The model under review builds one solid part; all positions refer to its coordinate system, in mm. A direction names the side the tool comes from. Round coordinates to 2 decimals unless told otherwise and drop trailing zeros. Order: outer loops, then holes, each group sorted by start corner. A loop starts at its lowest first (then second) coordinate and runs counter-clockwise, first axis right, second up. Notation, with made-up numbers: M 6.5,51.25 L 52.5,51.25 A18 ccw 52.5,70.25 Z; hole C 35,19.25 d7. An arc over 180 degrees is marked long. Answer as a JSON object with one key per item and string values. Group by question number.
1) Consider section C-C, the plane z = 94. Write out the cut boundary in (x, y), then the cut area to 3 significant figures.
2) Consider section B-B, the plane x = -5. Write out the cut boundary in (y, z), then the cut area to 3 significant figures.
3) Consider section A-A, the plane y = 1. Write out the cut boundary in (x, z).
4) The part is to be moulded in two halves that separate along X. For faces 3 (the flat face through (-35.466, 4, 50)), 4 (the flat face through (2, -27.251, 95)), 5 (the flat face through (-32, 5, 101.6)), say which applies: +X half, -X half, draft (parallel to the pull), parting line (faces both ways), or undercut.
5) To check wall thickness, follow line 1 (Y direction, x = -20, z = 91); line 2 (Z direction, x = 15.5, y = 18). State the ranges of each line that lie inside material, in increasing order.
6) For faces 1 (the flat face through (2, 42.599, 50)), 2 (the flat face through (2, 5, 88.9)), list the 3-axis set-ups (+Z, -Z, +X, -X, +Y, -Y) from which the entire face can be reached by the end or side of a thin tool; tool diameter is ignored.
7) Insertion check: pin 1 Ø2 at (x, y) = (7, -21) entering from +Z. The pin has a flat end and moves straight along its axis. Give the tip position at first contact, or say it passes through.
```python
from build123d import *

# Parameters (mm, degrees)
F0_W     = 76.2
F0_H     = 76.2
F1_DEPTH = 76.2
F2_DEPTH = 25.4
F3_W     = 63.5
F3_H     = 63.5000005424
F4_DEPTH = 12.7


with BuildPart() as f1:
    # F0 (on Top) → F1 (new body)
    with BuildSketch(Plane.XY):
        with Locations((2.6339268429, 4.4994018972)):
            Rectangle(F0_W, F0_H)
    extrude(amount=F1_DEPTH)

    # F2 (add): a face of the model
    f2_faces = [f1.faces().sort_by_distance(p)[0] for p in [
        (2.6339268429, 4.4994018972, 76.2),
    ]]
    extrude(f2_faces, amount=F2_DEPTH)

    # F3 (on face) → F4 (cut)
    with BuildSketch(Plane.XY.offset(101.6)):
        with Locations((2.6339268429, 4.4994021684)):
            Rectangle(F3_W, F3_H)
    extrude(amount=-F4_DEPTH, mode=Mode.SUBTRACT)


solid = f1.part
```
Results list:
{
 "1": {"outline": "M -35.47,-33.6 L 40.73,-33.6 L 40.73,42.6 L -35.47,42.6 Z; hole M -29.12,-27.25 L 34.38,-27.25 L 34.38,36.25 L -29.12,36.25 Z", "area": "1,770 mm^2"},
 "2": {"outline": "M -33.6,0 L 42.6,0 L 42.6,101.6 L 36.25,101.6 L 36.25,88.9 L -27.25,88.9 L -27.25,101.6 L -33.6,101.6 Z", "area": "6,940 mm^2"},
 "3": {"outline": "M -35.47,0 L 40.73,0 L 40.73,101.6 L 34.38,101.6 L 34.38,88.9 L -29.12,88.9 L -29.12,101.6 L -35.47,101.6 Z"},
 "4": {"face 3": "-X half", "face 4": "undercut", "face 5": "draft"},
 "5": {"line 1": "-33.6 to -27.25, 36.25 to 42.6", "line 2": "0 to 88.9"},
 "6": {"face 1": "+Z, -Z, +X, -X, +Y", "face 2": "+Z"},
 "7": {"pin 1": "z = 88.9"}
}
